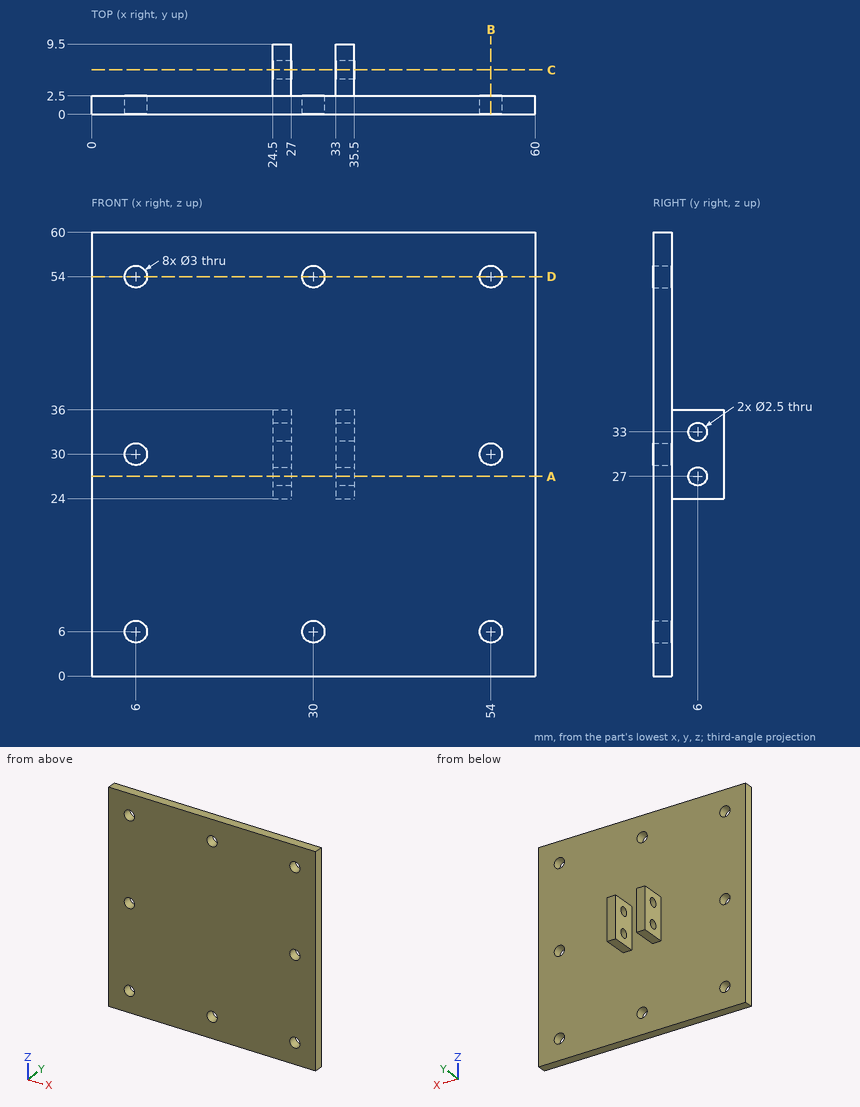
The drawing under review shows one solid part. Ordinate dimensions are in mm from its lowest x, y, z. Round coordinates to 2 decimals unless told otherwise and drop trailing zeros. Loops run counter-clockwise (first coordinate to the right, second up) from the corner with the lowest first, then second, coordinate; pieces in that order, holes last. Notation, with made-up numbers: (88.25, 24.5) - (133.25, 24.5) arc R29 cw to (133.25, 44.5) - close; hole circle Ø8 at (47.5, -3). An arc over 180 degrees is marked (long way). One line per question, with ' | ' between items.
Q1. Take a section at C-C (y = 6). Give the boundary of the cut face in (x, z).
Taken from the geometry:
outline: (24.5, 24) - (27, 24) - (27, 25.75) - (24.5, 25.75) - close; (24.5, 28.25) - (27, 28.25) - (27, 31.75) - (24.5, 31.75) - close; (24.5, 34.25) - (27, 34.25) - (27, 36) - (24.5, 36) - close; (33, 24) - (35.5, 24) - (35.5, 25.75) - (33, 25.75) - close; (33, 28.25) - (35.5, 28.25) - (35.5, 31.75) - (33, 31.75) - close; (33, 34.25) - (35.5, 34.25) - (35.5, 36) - (33, 36) - close
Q2. Take a section at B-B (x = 54). Give the boundary of the cut face in (y, z).
Taken from the geometry:
outline: (0, 0) - (2.5, 0) - (2.5, 4.5) - (0, 4.5) - close; (0, 7.5) - (2.5, 7.5) - (2.5, 28.5) - (0, 28.5) - close; (0, 31.5) - (2.5, 31.5) - (2.5, 52.5) - (0, 52.5) - close; (0, 55.5) - (2.5, 55.5) - (2.5, 60) - (0, 60) - close
Q3. Take a section at A-A (z = 27). Give the boundary of the cut face in (x, y).
Taken from the geometry:
outline: (0, 0) - (60, 0) - (60, 2.5) - (35.5, 2.5) - (35.5, 4.75) - (33, 4.75) - (33, 2.5) - (27, 2.5) - (27, 4.75) - (24.5, 4.75) - (24.5, 2.5) - (0, 2.5) - close; (24.5, 7.25) - (27, 7.25) - (27, 9.5) - (24.5, 9.5) - close; (33, 7.25) - (35.5, 7.25) - (35.5, 9.5) - (33, 9.5) - close
Q4. For line 1 along X through (y, z) = (0.6, 30); line 2 along X through (y, z) = (1, 6), list the stretches that pass through material, from the lowest coordinate up. Write a range as [from, to].
Taken from the geometry:
line 1: x = [0, 4.5], [7.5, 52.5], [55.5, 60] | line 2: x = [0, 4.5], [7.5, 28.5], [31.5, 52.5], [55.5, 60]
Q5. For pin 1 (5.5 mm diameter, centred on y = 7.5, z = 29, fed in from -X); pin 2 (4 mm diameter, centred on y = 6, z = 33, fed in from +X); pin 3 (3.5 mm diameter, centred on x = 6, z = 6, fed in from +Y), all flat-tipped, find the tip position at first contact; note any pin that passes through.
Taken from the geometry:
pin 1: stops at x = 24.5 | pin 2: stops at x = 35.5 | pin 3: stops at y = 2.5
Q6. Take a section at D-D (z = 54). Give the boundary of the cut face in (x, y).
Taken from the geometry:
outline: (0, 0) - (4.5, 0) - (4.5, 2.5) - (0, 2.5) - close; (7.5, 0) - (28.5, 0) - (28.5, 2.5) - (7.5, 2.5) - close; (31.5, 0) - (52.5, 0) - (52.5, 2.5) - (31.5, 2.5) - close; (55.5, 0) - (60, 0) - (60, 2.5) - (55.5, 2.5) - close
